CAD build for the part. Positions are in the model's coordinates, mm. Face numbers are marked on the shaded views. Give positions to 0.01 mm unless a question says otherwise; leave off trailing zeros. Order: outer loops, then holes, each group sorted by start corner. A loop starts at its lowest first (then second) coordinate and runs counter-clockwise, first axis right, second up. Notation, with made-up numbers: (81.5, -18.75) -> (112.5, -18.75) arc R10 cw to (112.5, -0.75) -> close; hole circle Ø6 at (62, -7). An arc over 180 degrees is marked (long way). Use one line per item in the form item = value. Start each with the question number.
1) Cut at A-A, the plane z = -15. Give the cut face in (x, y).
2) Probe line 1 (X direction, y = 15, z = -31.1); line 2 (X direction, y = 10, z = -30.8); line 3 (Y direction, x = 15, z = -31). List the from-to ranges inside material, lowest first.
3) Drop flat-ended pins along their axis: P1, Ø6.5, axis at x = 50, y = 15, coming from the +Z side; P2, Ø1, axis at x = 150, y = 40, coming from the +Z side; P3, Ø8, axis at x = 274.5, y = 54.5, coming from the +Z side; P4, Ø9, axis at x = 15, y = 50, coming from the -Z side. Give the stop position or say it passes through.
4) Mould opens along Y. For the marked faces 1, 2 and 3 say: pulls with the +Y half, pulls with the -Y half, needs draft (parallel to the pull), parting line crosses it, or undercut.
5) Cut at B-B, the plane x = 50. State how many separate pieces and enclosed holes the cut face has, and give its area (3 significant figures).
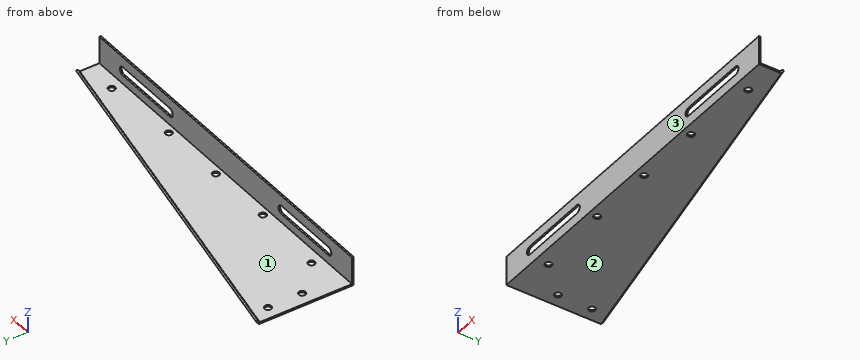
from build123d import *

# Parameters (mm, degrees)
BOSS_EXTRUDE1_DEPTH = 2
SKETCH3_W           = 430
SKETCH3_H           = 2
BOSS_EXTRUDE2_DEPTH = 30
CUT_EXTRUDE1_DEPTH  = 50
SKETCH7_R           = 4
CUT_EXTRUDE2_DEPTH  = 445.998876403
SKETCH8_R           = 4
CUT_EXTRUDE3_DEPTH  = 445.998876403
BOSS_EXTRUDE4_REACH = 466.157
FILLET3_R           = 1
FILLET4_R           = 1
SKETCH14_W          = 14.198164628
SKETCH14_H          = 140.679364316
CUT_EXTRUDE6_DEPTH  = 446.935341302


with BuildPart() as part:
    # Sketch2 → Boss-Extrude1 (new body)
    with BuildSketch(Plane.XY):
        Polygon((0, 0), (430, 0), (430, 25), (0, 110), align=None)
    boss_extrude1 = extrude(amount=BOSS_EXTRUDE1_DEPTH)

    # Sketch3 → Boss-Extrude2 (add)
    with BuildSketch(Plane(origin=(0, 0, 0), x_dir=(-1, 0, 0), z_dir=(0, 0, -1))):
        with Locations((-215, 1)):
            Rectangle(SKETCH3_W, SKETCH3_H)
    extrude(amount=BOSS_EXTRUDE2_DEPTH)

    # Sketch4 → Cut-Extrude1 (cut)
    with BuildSketch(Plane(origin=(0, 2, 0), x_dir=(1, 0, 0), z_dir=(0, 1, 0))):
        with BuildLine():
            Line((40, 20), (120, 20))
            ThreePointArc((120, 20), (125, 15), (120, 10))
            Line((120, 10), (40, 10))
            ThreePointArc((40, 10), (35, 15), (40, 20))
        make_face()
        with BuildLine():
            Line((390, 20), (310, 20))
            ThreePointArc((310, 20), (305, 15), (310, 10))
            Line((310, 10), (390, 10))
            ThreePointArc((390, 10), (395, 15), (390, 20))
        make_face()
    extrude(amount=-CUT_EXTRUDE1_DEPTH, mode=Mode.SUBTRACT)

    # Sketch7 → Cut-Extrude2 (cut, through all)
    with BuildSketch(Plane.XY.offset(2)):
        with Locations((15, 50)):
            Circle(SKETCH7_R)
        with Locations((50, 15)):
            Circle(SKETCH7_R)
        with Locations((390, 15)):
            Circle(SKETCH7_R)
        with Locations((15, 90)):
            Circle(SKETCH7_R)
    cut_extrude2 = extrude(amount=-CUT_EXTRUDE2_DEPTH, mode=Mode.SUBTRACT)

    # Sketch8 → Cut-Extrude3 (cut, through all)
    with BuildSketch(Plane.XY.offset(2)):
        with Locations((140, 10)):
            Circle(SKETCH8_R)
        with Locations((220, 10)):
            Circle(SKETCH8_R)
        with Locations((300, 10)):
            Circle(SKETCH8_R)
    cut_extrude3 = extrude(amount=-CUT_EXTRUDE3_DEPTH, mode=Mode.SUBTRACT)

    # Boss-Extrude4: up to this plane
    boss_extrude4_end = Plane(origin=(430, 0, 2), z_dir=(-1, 0, 0))
    # Sketch12 → Boss-Extrude4 (add, up to the surface)
    with BuildSketch(Plane(origin=(-20.926480156, 4.136629798, 0), x_dir=(0, 0, -1), z_dir=(0.9810169593645325, -0.19392195708368665, 0)), mode=Mode.PRIVATE) as boss_extrude4_sk1:
        with BuildLine():
            Line((2.668468057, 109.913216573), (0, 107.91186553))
            Line((0, 107.91186553), (-2, 107.91186553))
            Line((-2, 107.91186553), (-2, 108.91186553))
            Line((-2, 108.91186553), (1.468468057, 111.513216573))
            ThreePointArc((1.468468057, 111.513216573), (2.868468057, 111.313216573), (2.668468057, 109.913216573))
        make_face()
    boss_extrude4_tool1 = split(extrude(boss_extrude4_sk1.sketch, amount=BOSS_EXTRUDE4_REACH, mode=Mode.PRIVATE), bisect_by=boss_extrude4_end, keep=Keep.BOTH, mode=Mode.PRIVATE)
    boss_extrude4 = boss_extrude4_tool1.solids().sort_by_distance((0.341058, 111.725355, -0.613229))[0]
    add(boss_extrude4)

    # Fillet3
    fillet3_edges = [part.edges().sort_by_distance(p)[0] for p in [
        (215.096960979, 68.500183664, 2),
        (215, 67.5, 0),
    ]]
    fillet(fillet3_edges, radius=FILLET3_R)

    # Mirror1: Boss-Extrude1 across plane
    add(boss_extrude1.mirror(Plane(origin=(0, 0, -15), x_dir=(1, 0, 0), z_dir=(0, 0, -1))))

    # Mirror2: Boss-Extrude4 across plane
    add(boss_extrude4.mirror(Plane(origin=(0, 0, -15), x_dir=(1, 0, 0), z_dir=(0, 0, -1))))

    # Fillet4
    fillet4_edges = [part.edges().sort_by_distance(p)[0] for p in [
        (215, 67.5, -30),
        (215.096960979, 68.500183664, -32),
    ]]
    fillet(fillet4_edges, radius=FILLET4_R)

    # Sketch14 → Cut-Extrude6 (cut, through all)
    with BuildSketch(Plane.ZY):
        with Locations((1.254098972, 72.339682158)):
            Rectangle(SKETCH14_W, SKETCH14_H)
    extrude(amount=-CUT_EXTRUDE6_DEPTH, mode=Mode.SUBTRACT)

    # Mirror3: Cut-Extrude2, Cut-Extrude3 across plane
    add(cut_extrude2.mirror(Plane(origin=(0, 0, -15), x_dir=(1, 0, 0), z_dir=(0, 0, -1))), mode=Mode.SUBTRACT)
    add(cut_extrude3.mirror(Plane(origin=(0, 0, -15), x_dir=(1, 0, 0), z_dir=(0, 0, -1))), mode=Mode.SUBTRACT)


solid = part.part
Result:
q1.outline = (0, 0) -> (35, 0) -> (35, 2) -> (0, 2) -> close; (125, 0) -> (305, 0) -> (305, 2) -> (125, 2) -> close; (395, 0) -> (430, 0) -> (430, 2) -> (395, 2) -> close
q2.line_1 = 0 to 46, 54 to 386, 394 to 430
q2.line_2 = 0 to 136, 144 to 216, 224 to 296, 304 to 430
q2.line_3 = 0 to 46, 54 to 86, 94 to 108.82
q3.P1 = through
q3.P2 = -30
q3.P3 = -26.93
q3.P4 = -32
q4.face_1 = undercut
q4.face_2 = needs draft
q4.face_3 = pulls with the -Y half
q5.separate_pieces = 3
q5.enclosed_holes = 0
q5.area = 239 mm²
